```python
from build123d import *

# Parameters (mm, degrees)
SKETCH1_W      = 215.9
SKETCH1_H      = 25.4
SKETCH1_R      = 6.35
SKETCH1_R_2    = 7.874
EXTRUDE1_DEPTH = 1.524
FILLET1_R      = 5.08


with BuildPart() as part:
    # Sketch1 → Extrude1 (new, symmetric)
    with BuildSketch(Plane.XY):
        Rectangle(SKETCH1_W, SKETCH1_H)
        with Locations(Location((92.71, 0, 0), (0, 0, 180))):
            Circle(SKETCH1_R, mode=Mode.SUBTRACT)
        with Locations(Location((0, 0, 0), (0, 0, 180))):
            Circle(SKETCH1_R_2, mode=Mode.SUBTRACT)
        with Locations(Location((-92.71, 0, 0), (0, 0, 180))):
            Circle(SKETCH1_R, mode=Mode.SUBTRACT)
    extrude(amount=EXTRUDE1_DEPTH, both=True)

    # Fillet1
    fillet1_edges = [part.edges().sort_by_distance(p)[0] for p in [
        (-107.95, 12.7, 0),
        (107.95, 12.7, 0),
        (107.95, -12.7, 0),
        (-107.95, -12.7, 0),
    ]]
    fillet(fillet1_edges, radius=FILLET1_R)


solid = part.part
```
Design review of the part built by this model. Coordinates are the model's own, in mm. Give positions to 0.01 mm unless a question says otherwise; leave off trailing zeros. Order: outer loops, then holes, each group sorted by start corner. A loop starts at its lowest first (then second) coordinate and runs counter-clockwise, first axis right, second up. Notation, with made-up numbers: M 5.25,12.5 L 9.25,12.5 A5 ccw 9.25,19.5 Z; hole C -36.75,-14 d9. An arc over 180 degrees is marked long. One line per question, with ' | ' between items. Start each with the question number.
Q1. We need section C-C (z = -0.45). Write out the cut boundary in (x, y).
Q2. We need section D-D (x = -92.71). Write out the cut boundary in (y, z), plus the area to 3 significant figures.
Q3. We need section A-A (y = 0). Write out the cut boundary in (x, z), plus the area to 3 significant figures.
Q4. We need section B-B (x = 0). Write out the cut boundary in (y, z).
Q5. The part is to be moulded in two halves that separate along Y. For faces 1 (the face through (-106.501, -11.172, 0.021)), 2 (the face through (-2, 9, -1.524)), 3 (the face through (1.707, 7.687, -0.021)), 4 (the face through (-98.767, -1.907, -0.021)), say which applies: +Y half, -Y half, draft (parallel to the pull), parting line (faces both ways), or undercut.
Q6. For L1, parallel to Y at x = -92.71, z = -0.1; L2, parallel to Y at x = 0, z = 0; L3, parallel to X at y = -0.75, z = 0.9, list the stretches that pass through material, from the lowest coordinate up. Write a range as [from, to].
Returned:
1) outline: M -107.95,-7.62 A5.08 ccw -102.87,-12.7 L 102.87,-12.7 A5.08 ccw 107.95,-7.62 L 107.95,7.62 A5.08 ccw 102.87,12.7 L -102.87,12.7 A5.08 ccw -107.95,7.62 Z; hole C -92.71,0 d12.7; hole C 0,0 d15.75; hole C 92.71,0 d12.7
2) outline: M -12.7,-1.52 L -6.35,-1.52 L -6.35,1.52 L -12.7,1.52 Z; M 6.35,-1.52 L 12.7,-1.52 L 12.7,1.52 L 6.35,1.52 Z | area: 38.7 mm2
3) outline: M -107.95,-1.52 L -99.06,-1.52 L -99.06,1.52 L -107.95,1.52 Z; M -86.36,-1.52 L -7.87,-1.52 L -7.87,1.52 L -86.36,1.52 Z; M 7.87,-1.52 L 86.36,-1.52 L 86.36,1.52 L 7.87,1.52 Z; M 99.06,-1.52 L 107.95,-1.52 L 107.95,1.52 L 99.06,1.52 Z | area: 533 mm2
4) outline: M -12.7,-1.52 L -7.87,-1.52 L -7.87,1.52 L -12.7,1.52 Z; M 7.87,-1.52 L 12.7,-1.52 L 12.7,1.52 L 7.87,1.52 Z
5) face 1: -Y half | face 2: draft | face 3: undercut | face 4: undercut
6) L1: [-12.7, -6.35], [6.35, 12.7] | L2: [-12.7, -7.87], [7.87, 12.7] | L3: [-107.95, -99.02], [-86.4, -7.84], [7.84, 86.4], [99.02, 107.95]
